Check sheet for the drawn part. Datum: minimum x, y, z corner. Units: mm. A direction names the side the tool comes from. Coordinates: 2 decimals unless noted, no trailing zeros. Order: outer loops, then holes, each group sorted by start corner. A loop starts at its lowest first (then second) coordinate and runs counter-clockwise, first axis right, second up. Notation, with made-up numbers: (36, 9) - (48, 9) arc R27 ccw to (48, 41) - close; hole circle Ø10 at (-6.5, 59.5). An arc over 180 degrees is marked (long way). Return JSON: item names as keys, results as strings. Group by question number.
Item 1: Section check C-C on x = 12.5. Enter the section's corners in (y, z).
Item 2: Scan lines: probe 1 along X at (y, z) = (37, 2); probe 2 along Y at (x, z) = (28, 5.5). Record each from-to range of solid material in increasing order.
Item 3: Section check A-A on y = 38.5. Enter the section's corners in (x, z), then the cut area to 3 significant figures.
Item 4: Draft check along X on the marked faces 3, 4 and 5. Enter one of: pulls with the +X half, pulls with the -X half, needs draft (parallel to the pull), parting line crosses it, or undercut.
Item 5: Section check B-B on z = 1.75. Enter the section's corners in (x, y).
Item 6: Tool access check on the marked faces 1 and 2. Record the directions out of +Z, -Z, +X, -X, +Y, -Y that give a thin tool (end or side, any length) a straight path to the whole face; none if there is none.
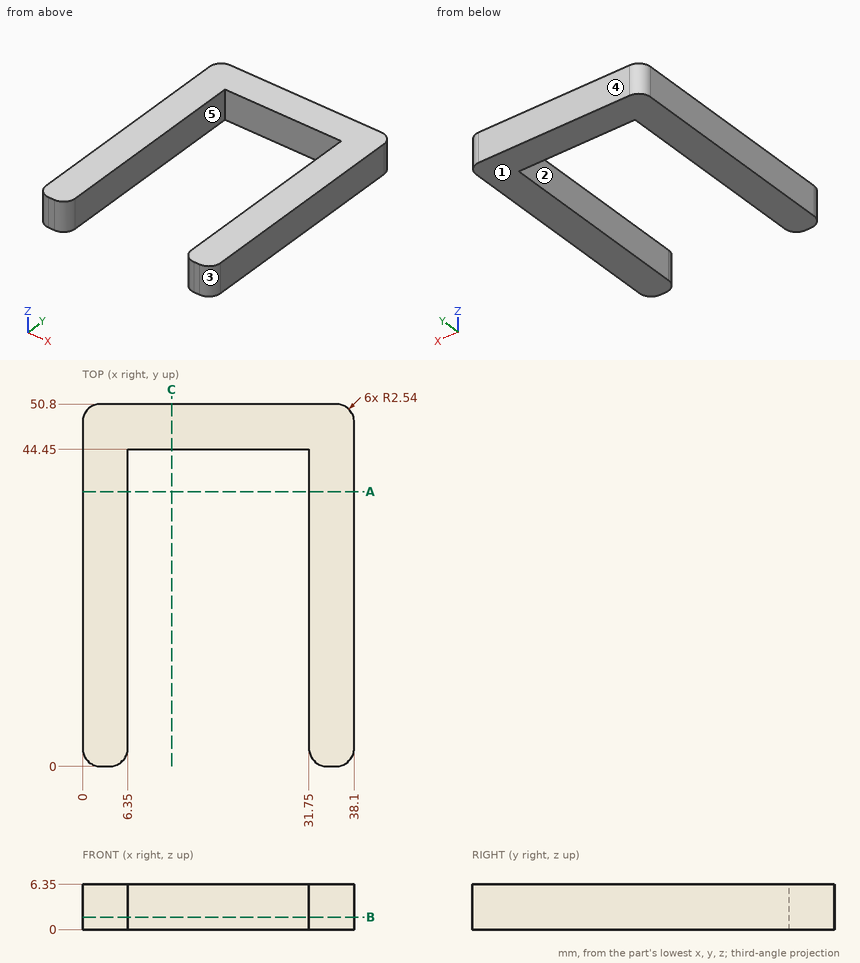
Computed:
{
 "1": {"outline": "(44.45, 0) - (50.8, 0) - (50.8, 6.35) - (44.45, 6.35) - close"},
 "2": {"probe 1": "x = 0 to 6.35, 31.75 to 38.1", "probe 2": "y = 44.45 to 50.8"},
 "3": {"outline": "(0, 0) - (6.35, 0) - (6.35, 6.35) - (0, 6.35) - close; (31.75, 0) - (38.1, 0) - (38.1, 6.35) - (31.75, 6.35) - close", "area": "80.6 mm²"},
 "4": {"face 3": "pulls with the +X half", "face 4": "needs draft", "face 5": "undercut"},
 "5": {"outline": "(0, 2.54) arc R2.54 ccw to (2.54, 0) - (3.81, 0) arc R2.54 ccw to (6.35, 2.54) - (6.35, 44.45) - (31.75, 44.45) - (31.75, 2.54) arc R2.54 ccw to (34.29, 0) - (35.56, 0) arc R2.54 ccw to (38.1, 2.54) - (38.1, 48.26) arc R2.54 ccw to (35.56, 50.8) - (2.54, 50.8) arc R2.54 ccw to (0, 48.26) - close"},
 "6": {"face 1": "-Z, +X, -X, +Y, -Y", "face 2": "+Z, -Z, -Y"}
}
